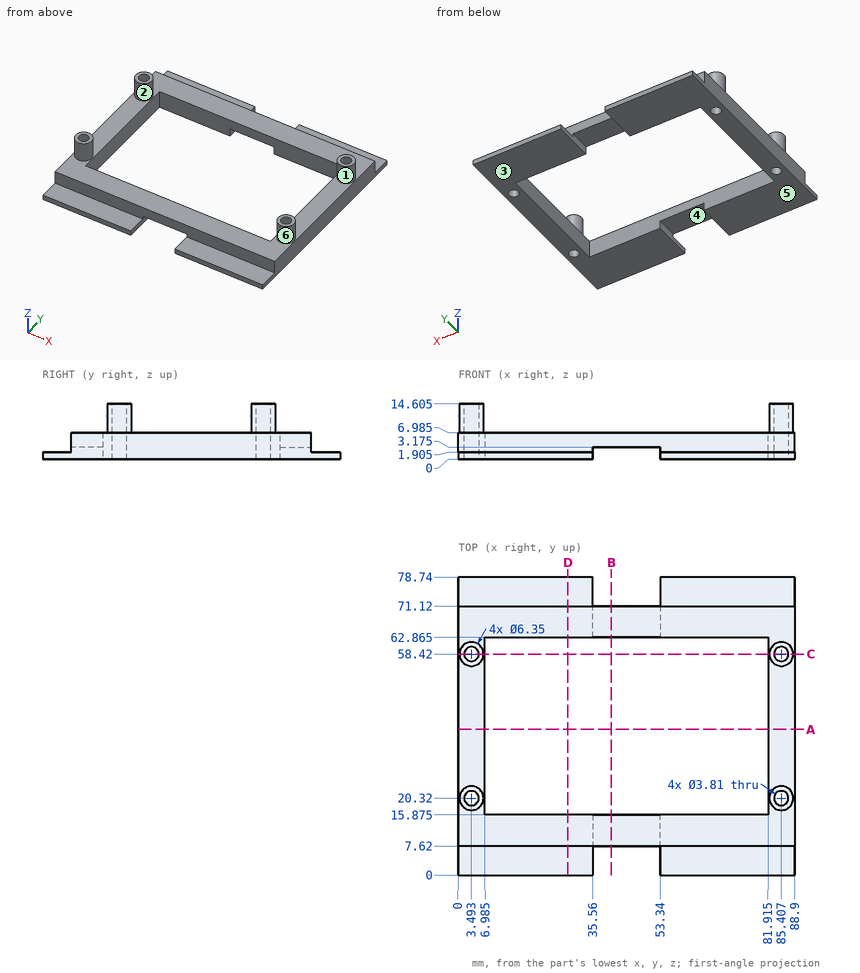
Answer from the drawing. Dimensions are ordinates in mm from the lowest x, y and z of the part. A direction names the side the tool comes from. Give positions to 0.01 mm unless a question says otherwise; leave off trailing zeros. Write each loop counter-clockwise with the first axis right and the second up, starting at its lowest first coordinate (ties: lowest second). Pieces come first, ordered by that corner, then holes. Notation, with made-up numbers: (13, 75.25) - (57, 75.25) arc R20 cw to (57, 100.25) - close; hole circle Ø9 at (34, 41.5). An arc over 180 degrees is marked (long way). Answer in a Markdown table with one row per item. Add a question column.
Item 1: Section A-A, the plane y = 38.5 is taken. Write down the section's boundary in (x, z) (1 decimal).
Item 2: Flat-ended cylindrical pins translate along their axes: P1, Ø8.5, axis at x = 79, y = 4, coming from the +Z side (1 decimal); P2, Ø2, axis at x = 57, z = 4.5, coming from the +Y side; P3, Ø6.5, axis at x = 47, y = 68, coming from the -Z side (1 decimal); P4, Ø5, axis at x = 78, y = 27.5, coming from the -Z side. Find the tip coordinate at first contact, or state that the pin passes through.
Item 3: Section C-C, the plane y = 58.42 is taken. Count the separate pieces of the cut face and the enclosed holes in it.
Item 4: Find the intervals of material crossed by L1, parallel to X at y = 20.5, z = 12.5 (1 decimal); L2, parallel to X at y = 69, z = 2; L3, parallel to X at y = 56, z = 4.25 (1 decimal), in increasing order.
Item 5: A tool of negligible diameter and unlimited length cuts with its end or side. For the marked faces 4, 5 and 6, from which of +Z, -Z, +X, -X, +Y, -Y can it reach the whole face along a straight path? Write none if from no direction.
Item 6: Section B-B, the plane x = 40.5 is taken. Write down the section's boundary in (y, z) (1 decimal).
Item 7: Determine the mould class of the marked faces 1, 2 and 3 for opening direction X: pulls with the +X half, pulls with the -X half, needs draft (parallel to the pull), parting line crosses it, or undercut.
Item 8: Section D-D, the plane x = 29 is taken. Write down the section's boundary in (y, z) (1 decimal).
Recorded:
| question | item | result |
|---|---|---|
| 1 | outline | (0, 0) - (7, 0) - (7, 7) - (0, 7) - close; (81.9, 0) - (88.9, 0) - (88.9, 7) - (81.9, 7) - close |
| 2 | P1 | stops at z = 7 |
| 2 | P2 | stops at y = 71.12 |
| 2 | P3 | stops at z = 3.2 |
| 2 | P4 | passes through |
| 3 | separate pieces | 4 |
| 3 | enclosed holes | 0 |
| 4 | L1 | x = 0.3 to 1.6, 5.4 to 6.7, 82.2 to 83.5, 87.3 to 88.6 |
| 4 | L2 | x = 0 to 35.56, 53.34 to 88.9 |
| 4 | L3 | x = 0 to 7, 81.9 to 88.9 |
| 5 | face 4 | -Z, +Y, -Y |
| 5 | face 5 | -Z, +X, -X, +Y, -Y |
| 5 | face 6 | +Z |
| 6 | outline | (7.6, 3.2) - (15.9, 3.2) - (15.9, 7) - (7.6, 7) - close; (62.9, 3.2) - (71.1, 3.2) - (71.1, 7) - (62.9, 7) - close |
| 7 | face 1 | undercut |
| 7 | face 2 | undercut |
| 7 | face 3 | needs draft |
| 8 | outline | (0, 0) - (15.9, 0) - (15.9, 7) - (7.6, 7) - (7.6, 1.9) - (0, 1.9) - close; (62.9, 0) - (78.7, 0) - (78.7, 1.9) - (71.1, 1.9) - (71.1, 7) - (62.9, 7) - close |
